Source: CAD feature listing. Evaluate the final solid. Frame: model axes, mm. Face numbers are marked on the shaded views. A direction names the side the tool comes from. Give positions to 0.01 mm unless a question says otherwise; leave off trailing zeros. Order: outer loops, then holes, each group sorted by start corner. A loop starts at its lowest first (then second) coordinate and runs counter-clockwise, first axis right, second up.
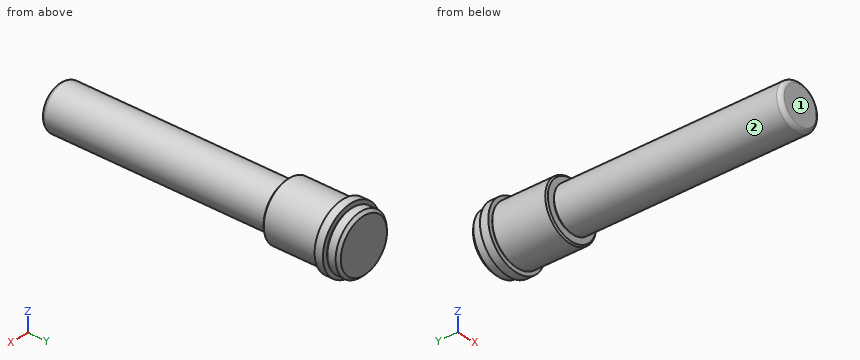
```python
from build123d import *


with BuildPart() as part:
    # Szkic1 → Obrót2 (revolve)
    with BuildSketch(Plane.XY):
        with BuildLine():
            Line((0, 188.802213019), (-19, 188.802213019))
            Line((-19, 188.802213019), (-21, 186.802213019))
            Line((-21, 186.802213019), (-21, 180.802213019))
            Line((-21, 180.802213019), (-20, 180.802213019))
            Line((-20, 180.802213019), (-20, 179.802213019))
            Line((-20, 179.802213019), (-23.5, 179.802213019))
            Line((-23.5, 179.802213019), (-23.5, 173.802213019))
            Line((-23.5, 173.802213019), (-21, 173.802213019))
            Line((-21, 173.802213019), (-20.3, 173.802213019))
            Line((-20.3, 173.802213019), (-20.3, 173.102213019))
            Line((-20.3, 173.102213019), (-21, 173.102213019))
            Line((-21, 173.102213019), (-21, 134.802213019))
            Line((-21, 134.802213019), (-20, 133.802213019))
            Line((-20, 133.802213019), (-15, 133.802213019))
            Line((-15, 133.802213019), (-15, 132.802213019))
            Line((-15, 132.802213019), (-16, 132.802213019))
            Line((-16, 132.802213019), (-16, -28.197786981))
            ThreePointArc((-16, -28.197786981), (-15.047167049, -30.067674085), (-13.278774205, -31.197786981))
            Line((-13.278774205, -31.197786981), (0, -31.197786981))
            Line((0, -31.197786981), (0, 188.802213019))
        make_face()
    revolve(axis=Axis((0, 188.802213019, 0), (0, -1, 0)))


solid = part.part
```
1) Pin query (flat end, axial travel): pin 1 (10 mm diameter, centred on y = 163, z = 5.5, fed in from +X); pin 2 (12 mm diameter, centred on x = -9, y = 147, fed in from -Z); pin 3 (1 mm diameter, centred on x = 5.5, y = 164.5, fed in from +Z). Return the tip coordinate at first contact, or that it passes through.
Report:
pin 1: stops at x = 20.99
pin 2: stops at z = -20.78
pin 3: stops at z = 20.4
2) Section query C-C, the plane y = 125.5. Return the cut outline in (x, z), and give its area (3 significant figures).
Report:
outline: circle Ø32 at (0, 0)
area: 804 mm2
3) Reachability of the marked faces 1 and 2 from +Z, -Z, +X, -X, +Y, -Y: full face, straight path, thin tool, end or side. Return the list, or none.
Report:
face 1: +Z, -Z, +X, -X, -Y
face 2: -Y
4) Material intervals for L1, parallel to Y at x = -4, z = -17.5; L2, parallel to Y at x = -16.5, z = 15; L3, parallel to Z at x = -0.5, y = -1, sorted ascending.
Report:
L1: y = 133.8 to 188.8
L2: y = 173.8 to 179.8
L3: z = -15.99 to 15.99
